The figure shows three views and two pictorial views of one solid part (mm, origin at its lowest corner). Answer the questions. A direction names the side the tool comes from. Coordinates: 2 decimals unless noted, no trailing zeros. Write each loop counter-clockwise with the first axis right and the second up, starting at its lowest first coordinate (ties: lowest second). Pieces come first, ordered by that corner, then holes. Notation, with made-up numbers: M -39,74 L -26,74 A23 ccw -26,106 Z; hole C 88.25,30.25 d3. An arc over 180 degrees is marked long. Answer as CSV lines item,"result".
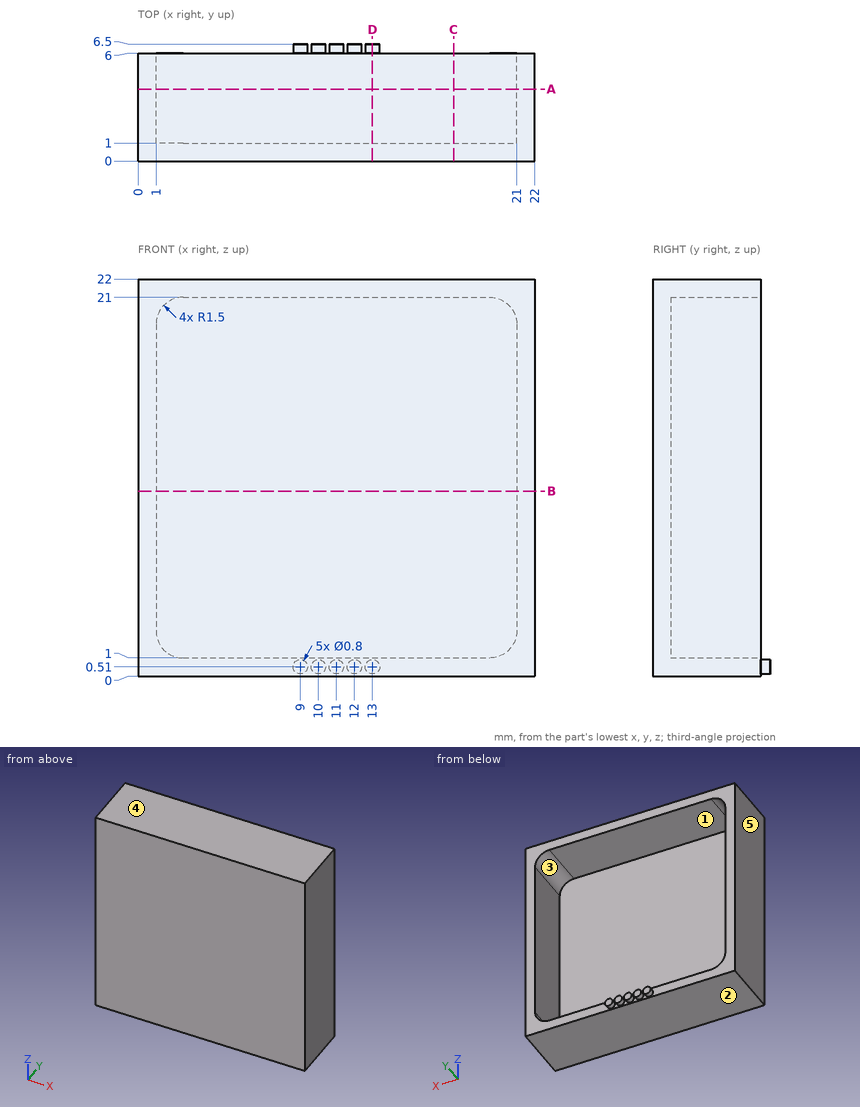
Q1. Straight lines are drawn through the part: line 1 (Z direction, x = 3.75, y = 1.75); line 2 (Y direction, x = 6.75, z = 11). For each, find the intervals that lie inside material, in ascending order.
Output:
line 1,"0 to 1, 21 to 22"
line 2,"0 to 1"
Q2. The mould has two halves that part along X. Classify the marked faces 3, 4 and 5: pulls with the +X half, pulls with the -X half, needs draft (parallel to the pull), parting line crosses it, or undercut.
Output:
face 3,"undercut"
face 4,"needs draft"
face 5,"pulls with the -X half"
Q3. For the marked faces 1 and 2, determine the directions among +Z, -Z, +X, -X, +Y, -Y from which every point of the face is accessible in a straight line to the end or side of a thin tool.
Output:
face 1,"+Y"
face 2,"-Z, +X, -X, +Y, -Y"
Q4. Find section C-C (x = 17.5). Give the vertices of the cut face in (y, z).
Output:
outline,"M 0,0 L 6,0 L 6,1 L 1,1 L 1,21 L 6,21 L 6,22 L 0,22 Z"
Q5. Find section D-D (x = 13). Give the vertices of the cut face in (y, z).
Output:
outline,"M 0,0 L 6,0 L 6,0.11 L 6.5,0.11 L 6.5,0.91 L 6,0.91 L 6,1 L 1,1 L 1,21 L 6,21 L 6,22 L 0,22 Z"
Q6. Find section A-A (y = 4). Give the vertices of the cut face in (x, z).
Output:
outline,"M 0,0 L 22,0 L 22,22 L 0,22 Z; hole M 1,2.5 A1.5 ccw 2.5,1 L 19.5,1 A1.5 ccw 21,2.5 L 21,19.5 A1.5 ccw 19.5,21 L 2.5,21 A1.5 ccw 1,19.5 Z"
Q7. A flat-ended cylindrical pin translates along its axis: pin 1 Ø8 at (x, z) = (11.5, 8) entering from +Y. Find the tip coordinate at first contact, or state that the pin passes through.
Output:
pin 1,"y = 1"
Q8. Find section B-B (z = 10.25). Give the vertices of the cut face in (x, y), and give its area (3 significant figures).
Output:
outline,"M 0,0 L 22,0 L 22,6 L 21,6 L 21,1 L 1,1 L 1,6 L 0,6 Z"
area,"32.0 mm2"
